Autodesk Inventor part; units mm, degrees
ref_plane "YZ Plane" through (0, 0, 0) normal (1, 0, 0) x (0, 1, 0)
ref_plane "XZ Plane" through (0, 0, 0) normal (0, 1, 0) x (-1, 0, 0)
ref_plane "XY Plane" through (0, 0, 0) normal (0, 0, 1) x (1, 0, 0)
sketch "Sketch1" plane through (0, 0, 0) normal (0, 1, 0) x (-1, 0, 0)
  circle A0 centre (0, 0) radius 1.465
  circle A1 centre (0, 0) radius 2.75
  line L0 (0.7073, -1.225) -> (-0.7073, -1.225)
  line L1 (-0.7073, -1.225) -> (-1.4145, 0)
  line L2 (-1.4145, 0) -> (-0.7073, 1.225)
  line L3 (-0.7073, 1.225) -> (0.7073, 1.225)
  line L4 (0.7073, 1.225) -> (1.4145, 0)
  line L5 (1.4145, 0) -> (0.7073, -1.225)
  dimension "d0" = 2.93
  dimension "d1" = 5.5
  dimension "d8" = 2.45
extrude "Extrusion1" add sketch "Sketch1" along normal blind 3 contours A0 | A1 | L0 L1 L2 L3 L4 L5
extrude "Extrusion2" add sketch "Sketch1" against normal blind 12 contours A0 | L0 L1 L2 L3 L4 L5
extrude "Extrusion3" cut sketch "Sketch1" against normal blind 2 from surface at 3 contours L0 L1 L2 L3 L4 L5
fillet "Fillet1" radius 0.5 1 edges at (2.75, 3, 0)
thread "Thread2"
equation "\"d4\" = length"
equation "\"length\" = 12"
properties part number "M3x16"
Part model, mm, in its own coordinate system. A direction names the side the tool comes from. Round coordinates to 2 decimals unless told otherwise and drop trailing zeros. Write each loop counter-clockwise with the first axis right and the second up, starting at its lowest first coordinate (ties: lowest second). Pieces come first, ordered by that corner, then holes.
Item 1: Two-plate mould, pull along X, no slides. Class faces 1 (the flat face through (0, 3, -1.5)), 2 (the cylindrical face through (0.32, -5.92, -1.43)), 3 (the flat face through (1.07, 2.01, 0.6)): +X half, -X half, draft (parallel to the pull), parting line (faces both ways), or undercut.
Results:
face 1: draft
face 2: parting line
face 3: undercut
Item 2: Cut at A-A, the plane x = 0. Give the cut face in (y, z) (3 decimals).
Results:
outline: (-12, -1.465) - (0, -1.465) - (0, -2.75) - (2.5, -2.75) arc R0.5 ccw to (3, -2.25) - (3, -1.225) - (1, -1.225) - (1, 1.225) - (3, 1.225) - (3, 2.25) arc R0.5 ccw to (2.5, 2.75) - (0, 2.75) - (0, 1.465) - (-12, 1.465) - close
Item 3: Cut at B-B, the plane y = -4.5. Give the cut face in (x, z) (3 decimals), plus the area to 3 significant figures.
Results:
outline: circle Ø2.93 at (0, 0)
area: 6.74 mm2
Item 4: Drop flat-ended pins along their axis: pin 1 Ø1.5 at (y, z) = (-10, 0.5) entering from -X (3 decimals); pin 2 Ø1 at (y, z) = (-2.5, -1) entering from +X; pin 3 Ø3 at (y, z) = (-1, -1.5) entering from -X. Give the stop position or say it passes through.
Results:
pin 1: stops at x = -1.465
pin 2: stops at x = 1.38
pin 3: stops at x = -2.72
Item 5: Which spindle directions (+Z, -Z, +X, -X, +Y, -Y) get a long thin tool onto all of the face, cutting with end or side? Do faces 4 (the flat face through (-1.2, 0, -1.2)), 5 (the flat face through (0, -12, 0)), 6 (the flat face through (-1.07, 2.01, -0.6)). Say none if no direction does.
Results:
face 4: -Y
face 5: +Z, -Z, +X, -X, -Y
face 6: +Y
Item 6: Probe L1, parallel to Y at x = -0.7, z = 1; L2, parallel to Y at x = 1.5, z = -0.75; L3, parallel to Z at x = -0.8, y = -7. List the from-to ranges inside material, lowest first.
Results:
L1: y = -12 to 1
L2: y = 0 to 3
L3: z = -1.23 to 1.23
